```python
from build123d import *

# Parameters (mm, degrees)
BOSS_EXTRUDE1_DEPTH         = 6.35
FILLET3_R                   = 3.175
F_10_CLEARANCE_HOLE1_D      = 5.1054
F_1_4_0_25_DIAMETER_HOLE1_D = 6.35
FILLET2_R                   = 3.175
F_10_24_TAPPED_HOLE1_D      = 3.7973
BOSS_EXTRUDE2_START         = -3.175
BOSS_EXTRUDE2_DEPTH         = 3.175
CUT_EXTRUDE1_DEPTH          = 7.35


with BuildPart() as part:
    # Sketch1 → Boss-Extrude1 (new body)
    with BuildSketch(Plane(origin=(0, 0, 0), x_dir=(1, 0, 0), z_dir=(0, 1, 0))):
        with BuildLine():
            Line((0, -7.9375), (19.05, -7.9375))
            ThreePointArc((19.05, -7.9375), (22.439261793, -8.697478788), (25.179511411, -10.831886268))
            Line((25.179511411, -10.831886268), (47.845488589, -38.380613732))
            ThreePointArc((47.845488589, -38.380613732), (56.653703924, -40.809343918), (61.9125, -33.3375))
            Line((61.9125, -33.3375), (61.9125, 14.2875))
            ThreePointArc((61.9125, 14.2875), (58.399282876, 20.877615878), (50.969601787, 21.634028965))
            Line((50.969601787, 21.634028965), (16.044601787, 7.346528965))
            ThreePointArc((16.044601787, 7.346528965), (13.502817622, 5.677382664), (11.775161084, 3.175))
            Line((11.775161084, 3.175), (7.274838916, 3.175))
            ThreePointArc((7.274838916, 3.175), (6.75922379, 4.161345937), (6.110713691, 5.065874499))
            Line((6.110713691, 5.065874499), (-18.894457111, 35.228374499))
            ThreePointArc((-18.894457111, 35.228374499), (-23.603599947, 37.97527834), (-28.973920802, 37.036576643))
            Line((-28.973920802, 37.036576643), (-67.46875, 14.811576643))
            ThreePointArc((-67.46875, 14.811576643), (-71.279874161, 6.363503718), (-64.484525706, 0.061294354))
            Line((-64.484525706, 0.061294354), (-0.984525706, -7.876205646))
            ThreePointArc((-0.984525706, -7.876205646), (-0.493215942, -7.922161592), (0, -7.9375))
        make_face()
        with BuildLine():
            Line((27.252413672, 1.640330855), (52.3875, -28.909406206))
            Line((52.3875, -28.909406206), (52.3875, 6.510370067))
            ThreePointArc((52.3875, 6.510370067), (49.550717124, 7.697384122), (47.377980705, 9.873517369))
            Line((47.377980705, 9.873517369), (27.252413672, 1.640330855))
        make_face(mode=Mode.SUBTRACT)
        with BuildLine():
            Line((-49.23043706, 7.753658904), (-11.734122555, 3.066619591))
            ThreePointArc((-11.734122555, 3.066619591), (-8.556248755, 4.690794106), (-8.896026797, 8.243451649))
            Line((-8.896026797, 8.243451649), (-21.263790491, 23.162072897))
            ThreePointArc((-21.263790491, 23.162072897), (-26.406741657, 22.34972166), (-30.946612893, 24.899119705))
            Line((-30.946612893, 24.899119705), (-50.424126778, 13.65377182))
            ThreePointArc((-50.424126778, 13.65377182), (-51.948576442, 10.27454265), (-49.23043706, 7.753658904))
        make_face(mode=Mode.SUBTRACT)
    extrude(amount=BOSS_EXTRUDE1_DEPTH)

    # Fillet3
    fillet3_edges = [part.edges().sort_by_distance(p)[0] for p in [
        (47.377980705, 3.175, -9.873517369),
        (27.252413672, 3.175, -1.640330855),
        (52.3875, 3.175, 28.909406206),
        (52.3875, 3.175, -6.510370067),
        (-21.263790491, 3.175, -23.162072897),
        (-30.946612893, 3.175, -24.899119705),
    ]]
    fillet(fillet3_edges, radius=FILLET3_R)

    # #10 Clearance Hole1 (through all)
    with Locations(Plane(origin=(0, 6.35, 0), x_dir=(1, 0, 0), z_dir=(0, 1, 0))):
        with Locations((0, 0), (19.05, 0)):
            Hole(F_10_CLEARANCE_HOLE1_D / 2)

    # 1/4 (0.25) Diameter Hole1 (through all)
    with Locations(Plane(origin=(0, 6.35, 0), x_dir=(1, 0, 0), z_dir=(0, 1, 0))):
        with Locations((53.975, 14.2875), (-63.5, 7.9375)):
            Hole(F_1_4_0_25_DIAMETER_HOLE1_D / 2)

    # Fillet2
    fillet2_edges = [part.edges().sort_by_distance(p)[0] for p in [
        (7.274838916, 3.175, -3.175),
        (11.775161084, 3.175, -3.175),
    ]]
    fillet(fillet2_edges, radius=FILLET2_R)

    # #10-24 Tapped Hole1 (through all)
    with Locations(Plane(origin=(0, 6.35, 0), x_dir=(1, 0, 0), z_dir=(0, 1, 0))):
        with Locations((53.975, -33.3375), (-25.005170802, 30.1625)):
            Hole(F_10_24_TAPPED_HOLE1_D / 2)

    # Sketch8 → Boss-Extrude2 (add)
    with BuildSketch(Plane(origin=(0, 6.35, 0), x_dir=(1, 0, 0), z_dir=(0, 1, 0)).offset(BOSS_EXTRUDE2_START)):
        with BuildLine():
            Line((39.110559377, -27.763988542), (47.845488589, -38.380613732))
            ThreePointArc((47.845488589, -38.380613732), (56.653703924, -40.809343918), (61.9125, -33.3375))
            Line((61.9125, -33.3375), (61.9125, -19.589346715))
            ThreePointArc((61.9125, -19.589346715), (59.332407848, -48.281187836), (39.110559377, -27.763988542))
        make_face()
        with BuildLine():
            Line((-28.973920802, 37.036576643), (-40.880170802, 30.1625))
            ThreePointArc((-40.880170802, 30.1625), (-22.202029092, 45.78805668), (-10.120105094, 24.644307915))
            Line((-10.120105094, 24.644307915), (-18.894457111, 35.228374499))
            ThreePointArc((-18.894457111, 35.228374499), (-23.603599947, 37.97527834), (-28.973920802, 37.036576643))
        make_face()
    extrude(amount=-BOSS_EXTRUDE2_DEPTH)

    # Sketch9 → Cut-Extrude1 (cut, through all)
    with BuildSketch(Plane(origin=(0, 6.35, 0), x_dir=(1, 0, 0), z_dir=(0, 1, 0))):
        with BuildLine():
            Line((6.110713691, 5.065874499), (-10.120105094, 24.644307915))
            ThreePointArc((-10.120105094, 24.644307915), (-22.202029092, 45.78805668), (-40.880170802, 30.1625))
            Line((-40.880170802, 30.1625), (-67.46875, 14.811576643))
            ThreePointArc((-67.46875, 14.811576643), (-71.279874161, 6.363503718), (-64.484525706, 0.061294354))
            Line((-64.484525706, 0.061294354), (-0.984525706, -7.876205646))
            ThreePointArc((-0.984525706, -7.876205646), (-6.960158794, 3.815769361), (6.110713691, 5.065874499))
        make_face()
    extrude(amount=-CUT_EXTRUDE1_DEPTH, mode=Mode.SUBTRACT)


solid = part.part
```
The listing builds one solid part. Answer for the finished solid, in the listing's coordinates (mm). A direction names the side the tool comes from. Give positions to 0.01 mm unless a question says otherwise; leave off trailing zeros. Write each loop counter-clockwise with the first axis right and the second up, starting at its lowest first coordinate (ties: lowest second). Pieces come first, ordered by that corner, then holes. Notation, with made-up numbers: (-23, -12) - (4, -12) arc R31 cw to (4, 20) - close; hole circle Ø1 at (36.5, 84.5). An arc over 180 degrees is marked (long way). Use one line per item in the form item = value. Start each with the question number.
1) The mould has two halves that part along Z. Classify faces 4 (the face through (50.23, 3.22, 23.06)), 5 (the face through (11.419, 3.219, -3.546)), 6 (the face through (58, 3.175, 41)): pulls with the +Z half, pulls with the -Z half, needs draft (parallel to the pull), parting line crosses it, or undercut.
2) Find section C-C on x = 44. Determine the outline of the cut face in (y, z) (3 decimals).
3) Find section B-B on z = 14. Determine the outline of the cut face in (x, y).
4) A tool of negligible diameter and unlimited length cuts with its end or side. For faces 1 (the face through (7.631, 3.219, -3.546)), 2 (the face through (61.912, 3, 5)), 3 (the face through (51.91, 3.22, -5.92)), from which of +Z, -Z, +X, -X, +Y, -Y can it reach the whole face along a straight path? Write none if from no direction.
5) Consider line 1 along Z through (x, y) = (0, 4.5); line 2 along Z through (x, y) = (9, 0.75); line 3 along X through (y, z) = (6, 1). Determine where each line is inside the solid, lowest interval first. Write a range as from..to.
6) Find section D-D on z = 0. Determine the outline of the cut face in (x, y).
7) Find section A-A on y = 5.5. Count the separate pieces of the cut face and the enclosed holes in it, plus the area to 3 significant figures.
8) A flat-ended cylindrical pin translates along its axis: pin 1 Ø1 at (y, z) = (1, 20) entering from -X. Find the tip coordinate at first contact, or state that the pin passes through.
Geometry results:
q1.face_4 = undercut
q1.face_5 = pulls with the -Z half
q1.face_6 = needs draft
q2.outline = (0, -18.783) - (6.35, -18.783) - (6.35, -8.492) - (0, -8.492) - close; (0, 18.715) - (6.35, 18.715) - (6.35, 33.707) - (3.175, 33.707) - (3.175, 45.687) - (0, 45.687) - close
q3.outline = (27.79, 0) - (40.12, 0) - (40.12, 6.35) - (27.79, 6.35) - close; (52.39, 0) - (61.91, 0) - (61.91, 6.35) - (52.39, 6.35) - close
q4.face_1 = -Z, +Y, -Y
q4.face_2 = -Z, +X, +Y
q4.face_3 = +Y, -Y
q5.line_1 = -7.94..-2.55, 2.55..7.94
q5.line_2 = -3.18..7.94
q5.line_3 = -7.87..-2.35, 2.35..16.7, 21.4..29.56, 52.39..61.91
q6.outline = (-7.94, 0) - (-2.55, 0) - (-2.55, 6.35) - (-7.94, 6.35) - close; (2.55, 0) - (16.5, 0) - (16.5, 6.35) - (2.55, 6.35) - close; (21.6, 0) - (29.28, 0) - (29.28, 6.35) - (21.6, 6.35) - close; (52.39, 0) - (61.91, 0) - (61.91, 6.35) - (52.39, 6.35) - close
q7.separate_pieces = 1
q7.enclosed_holes = 5
q7.area = 1,690 mm2
q8.pin_1 = 32.31
